from build123d import *
from build123d.topology import SkipClean

# Parameters (mm, degrees)
SKETCH_1_R          = 2.5
EXTRUDE_1_DEPTH     = 10
SKETCH_2_W          = 2
SKETCH_2_H          = 10
CUT_EXTRUDE_1_DEPTH = 10
SKETCH_3_R          = 1.5
CUT_EXTRUDE_2_DEPTH = 40.698866483
CHAMFER_1_SIZE      = 0.5
FILLET_1_R          = 1


with BuildPart() as part:
    # 草图1 → 凸台-拉伸1 (new body)
    with BuildSketch(Plane.XY):
        with BuildLine():
            Line((0, 0), (0, 8))
            ThreePointArc((0, 8), (-5, 13), (0, 18))
            Line((0, 18), (0, 24))
            Line((0, 24), (-2.5, 24))
            Line((-2.5, 24), (-17.395659833, 17.081234348))
            ThreePointArc((-17.395659833, 17.081234348), (-19.979326925, 12.569151657), (-16.582987314, 8.632261629))
            Line((-16.582987314, 8.632261629), (-10, 7))
            Line((-10, 7), (-10, 0))
            Line((-10, 0), (0, 0))
        make_face()
        with Locations((-15.5, 13)):
            Circle(SKETCH_1_R, mode=Mode.SUBTRACT)
    extrude_1 = extrude(amount=EXTRUDE_1_DEPTH)

    # 镜向1: 凸台-拉伸1 across plane
    with SkipClean():  # the faces are left unmerged after this step: merging them gives an invalid solid
        add(extrude_1.mirror(Plane(origin=(0, 18, 10), x_dir=(0, 0, 1), z_dir=(-1, 0, 0))))

    # 草图2 → 切除-拉伸1 (cut)
    with BuildSketch(Plane.XZ):
        with Locations((0, 5)):
            Rectangle(SKETCH_2_W, SKETCH_2_H)
    extrude(amount=-CUT_EXTRUDE_1_DEPTH, mode=Mode.SUBTRACT)

    # 草图3 → 切除-拉伸2 (cut, through all)
    with BuildSketch(Plane(origin=(10, 0, 0), x_dir=(0, 0, -1), z_dir=(1, 0, 0))):
        with Locations((-5, 3)):
            Circle(SKETCH_3_R)
    extrude(amount=-CUT_EXTRUDE_2_DEPTH, mode=Mode.SUBTRACT)

    # 倒角1
    chamfer_1_edges = [part.edges().sort_by_distance(p)[0] for p in [
        (-18, 13, 0),
        (-18, 13, 10),
        (18, 13, 10),
        (18, 13, 0),
        (0, 18, 0),
        (0, 18, 10),
        (-10, 3, 6.5),
    ]]
    chamfer(chamfer_1_edges, length=CHAMFER_1_SIZE)

    # 圆角1
    fillet_1_edges = [part.edges().sort_by_distance(p)[0] for p in [
        (-10, 0, 5),
        (-2.5, 24, 5),
        (10, 0, 5),
        (2.5, 24, 5),
    ]]
    fillet(fillet_1_edges, radius=FILLET_1_R - 0.0001)  # a hair under: the kernel refuses the full size


solid = part.part
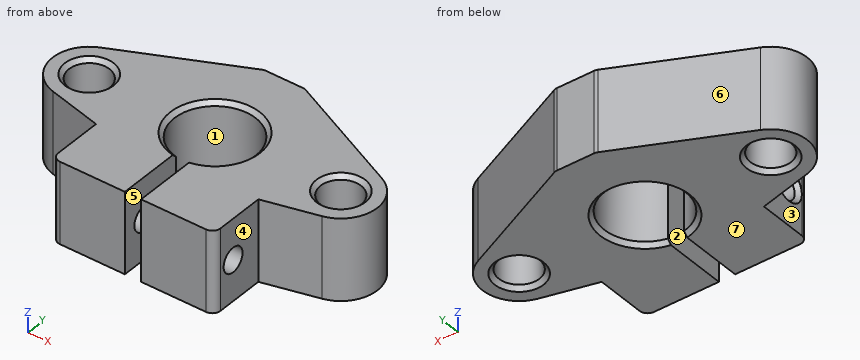
The listing builds one solid part. Answer for the finished solid, in the listing's coordinates (mm). Face numbers are marked on the shaded views. A direction names the side the tool comes from. Round coordinates to 2 decimals unless told otherwise and drop trailing zeros. Order: outer loops, then holes, each group sorted by start corner. A loop starts at its lowest first (then second) coordinate and runs counter-clockwise, first axis right, second up. Notation, with made-up numbers: (14, -36.5) -> (23, -36.5) arc R24 cw to (23, -21.5) -> close; hole circle Ø11 at (-23, 69). An arc over 180 degrees is marked (long way). Put each result on its own line as item: value.
Q1. Determine the mould class of the marked faces 5, 6 and 7 for opening direction X: pulls with the +X half, pulls with the -X half, needs draft (parallel to the pull), parting line crosses it, or undercut.
Results list:
face 5: undercut
face 6: pulls with the -X half
face 7: needs draft
Q2. Section B-B, the plane z = 2 is taken. Write down the section's boundary in (x, y).
Results list:
outline: (-17.4, 17.08) arc R4.5 ccw to (-16.58, 8.63) -> (-10, 7) -> (-10, 1) arc R1 ccw to (-9, 0) -> (-1, 0) -> (-1, 8.1) arc R5 cw (long way) to (1, 8.1) -> (1, 0) -> (9, 0) arc R1 ccw to (10, 1) -> (10, 7) -> (16.58, 8.63) arc R4.5 ccw to (17.4, 17.08) -> (2.7, 23.91) arc R1 ccw to (2.28, 24) -> (-2.28, 24) arc R1 ccw to (-2.7, 23.91) -> close; hole circle Ø5 at (-15.5, 13); hole circle Ø5 at (15.5, 13)
Q3. Which of the six approach directions +Z, -Z, +X, -X, +Y, -Y give full straight-line access (tool end or side, diameter ignored) to the marked faces 1, 2, 3 and 4?
Results list:
face 1: +Z, -Z
face 2: +Z, -Z, -Y
face 3: +Z, -Z, -X, -Y
face 4: +Z, -Z, +X, -Y
Q4. Consider line 1 along Y through (x, z) = (-4, 5); line 2 along X through (y, z) = (4.25, 0.75); line 3 along Y through (x, z) = (7.25, 5). Determine where each line is inside the solid, lowest interval first.
Results list:
line 1: 0 to 1.5, 4.5 to 10, 16 to 23.3
line 2: -10 to -1, 1 to 10
line 3: 0 to 1.5, 4.5 to 21.79
Q5. Each of these flat-tipped pins is pushed along its axis until it touches: P1, Ø13, axis at x = 0, y = 13, coming from the +Z side; P2, Ø5, axis at y = 3, z = 5, coming from the +X side; P3, Ø3, axis at x = 15, z = 1, coming from the -Y side; P4, Ø6, axis at x = 0.5, y = 13.5, coming from the +Z side. Where does it stop, or does it pass through?
Results list:
P1: z = 10
P2: x = 10
P3: y = 7.87
P4: through
Q6. Section A-A, the plane z = 5 is taken. Count the separate pieces of the cut face and the enclosed holes in it, and give its area (3 significant figures).
Results list:
separate pieces: 3
enclosed holes: 2
area: 457 mm^2
Q7. Section D-D, the plane x = -15.5 is taken. Write down the section's boundary in (y, z).
Results list:
outline: (8.36, 0) -> (10, 0) -> (10.5, 0.5) -> (10.5, 9.5) -> (10, 10) -> (8.36, 10) -> close; (15.5, 0.5) -> (16, 0) -> (17.96, 0) -> (17.96, 10) -> (16, 10) -> (15.5, 9.5) -> close
Q8. Section C-C, the plane y = 6 is taken. Write down the section's boundary in (x, z).
Results list:
outline: (-10, 0) -> (-1, 0) -> (-1, 10) -> (-10, 10) -> close; (1, 0) -> (10, 0) -> (10, 10) -> (1, 10) -> close
